The listing builds one solid part. Answer for the finished solid, in the listing's coordinates (mm). Face numbers are marked on the shaded views. Give positions to 0.01 mm unless a question says otherwise; leave off trailing zeros. Loops run counter-clockwise (first coordinate to the right, second up) from the corner with the lowest first, then second, coordinate; pieces in that order, holes last. Notation, with made-up numbers: M 36.25,-28.5 L 70.25,-28.5 A8 cw 70.25,-13.5 Z; hole C -17.75,35.25 d9. An arc over 180 degrees is marked long. One line per item, written item: value. Start each with the question number.
Q1. Flat-ended cylindrical pins translate along their axes: pin 1 (2 mm diameter, centred on x = 2, y = 2, fed in from +Z); pin 2 (4 mm diameter, centred on y = 5.5, z = 50.5, fed in from -X); pin 3 (4 mm diameter, centred on x = 5, z = 42, fed in from -Y); pin 4 (2 mm diameter, centred on y = 5.25, z = 51, fed in from -X). Find the tip coordinate at first contact, or state that the pin passes through.
Q2. The mould has two halves that part along X. Classify the marked faces 1, 2 and 3: +X half, -X half, draft (parallel to the pull), parting line (faces both ways), or undercut.
Q3. Consider L1, parallel to Z at x = 6.85, y = 5.25; L2, parallel to Z at x = 8, y = 2; L3, parallel to Y at x = 7.2, z = 91. Determine where each line is inside the solid, lowest interval first.
Q4. A cutting plane is placed at C-C, the plane z = 64.5. Determine the outline of the cut face in (x, y).
Q5. A cutting plane is placed at A-A, the plane z = 31. Determine the outline of the cut face in (x, y).
Q6. A cutting plane is placed at B-B, the plane x = 5.25. State how many separate pieces and enclosed holes the cut face has, and give its area (3 significant figures).
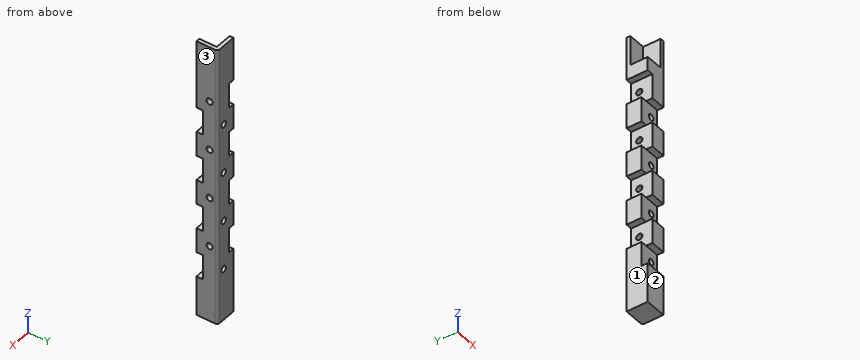
from build123d import *

# Parameters (mm, degrees)
SKETCH_W               = 8.5
SKETCH_H               = 8.5
PAD_DEPTH              = 113.5
SKETCH001_W            = 10
SKETCH001_H            = 10
POCKET_DEPTH           = 2.5
LINEARPATTERN_COUNT    = 4
LINEARPATTERN_PITCH    = 20
SKETCH002_W            = 10
SKETCH002_H            = 10
POCKET001_DEPTH        = 2.5
LINEARPATTERN001_COUNT = 4
LINEARPATTERN001_PITCH = 20
FILLET_R               = 1
SKETCH003_R            = 1.25
POCKET002_DEPTH        = 6.001
LINEARPATTERN002_COUNT = 4
LINEARPATTERN002_PITCH = 20
SKETCH004_R            = 1.25
POCKET003_DEPTH        = 6.001
LINEARPATTERN003_COUNT = 4
LINEARPATTERN003_PITCH = 20
SKETCH005_W            = 8.5
SKETCH005_H            = 8.5
POCKET004_DEPTH        = 12


with BuildPart() as part:
    # Sketch → Pad (new body)
    with BuildSketch(Plane.XY):
        with Locations((4.25, 4.25)):
            Rectangle(SKETCH_W, SKETCH_H)
    extrude(amount=PAD_DEPTH)

    # Sketch001 → Pocket (cut)
    with BuildSketch(Plane.XZ):
        with Locations((4.410969, 21)):
            Rectangle(SKETCH001_W, SKETCH001_H)
    pocket = extrude(amount=-POCKET_DEPTH, mode=Mode.SUBTRACT)

    # LinearPattern: Pocket ×4
    with Locations(*[(0, 0, i * LINEARPATTERN_PITCH) for i in range(1, LINEARPATTERN_COUNT)]):
        add(pocket, mode=Mode.SUBTRACT)

    # Sketch002 → Pocket001 (cut)
    with BuildSketch(Plane(origin=(0, 0, 0), x_dir=(0, -1, 0), z_dir=(-1, 0, 0))):
        with Locations((-4.326825, 31)):
            Rectangle(SKETCH002_W, SKETCH002_H)
    pocket001 = extrude(amount=-POCKET001_DEPTH, mode=Mode.SUBTRACT)

    # LinearPattern001: Pocket001 ×4
    with Locations(*[(0, 0, i * LINEARPATTERN001_PITCH) for i in range(1, LINEARPATTERN001_COUNT)]):
        add(pocket001, mode=Mode.SUBTRACT)

    # Fillet
    fillet_edges = [part.edges().sort_by_distance(p)[0] for p in [
        (8.5, 8.5, 56.75),
    ]]
    fillet(fillet_edges, radius=FILLET_R)

    # Sketch003 → Pocket002 (cut, through all)
    with BuildSketch(Plane.XZ.offset(-2.5)):
        with Locations((5.25, 21)):
            Circle(SKETCH003_R)
    pocket002 = extrude(amount=-POCKET002_DEPTH, mode=Mode.SUBTRACT)

    # LinearPattern002: Pocket002 ×4
    with Locations(*[(0, 0, i * LINEARPATTERN002_PITCH) for i in range(1, LINEARPATTERN002_COUNT)]):
        add(pocket002, mode=Mode.SUBTRACT)

    # Sketch004 → Pocket003 (cut, through all)
    with BuildSketch(Plane(origin=(2.5, 0, 0), x_dir=(0, -1, 0), z_dir=(-1, 0, 0))):
        with Locations((-5.25, 31)):
            Circle(SKETCH004_R)
    pocket003 = extrude(amount=-POCKET003_DEPTH, mode=Mode.SUBTRACT)

    # LinearPattern003: Pocket003 ×4
    with Locations(*[(0, 0, i * LINEARPATTERN003_PITCH) for i in range(1, LINEARPATTERN003_COUNT)]):
        add(pocket003, mode=Mode.SUBTRACT)

    # Sketch005 → Pocket004 (cut)
    with BuildSketch(Plane.XY.offset(113.5)):
        with Locations((2.75, 2.75)):
            Rectangle(SKETCH005_W, SKETCH005_H)
    extrude(amount=-POCKET004_DEPTH, mode=Mode.SUBTRACT)


solid = part.part
Answer block:
1. pin 1: z = 101.5
1. pin 2: x = 2.5
1. pin 3: y = 2.5
1. pin 4: through
2. face 1: -X half
2. face 2: draft
2. face 3: +X half
3. L1: 0 to 29.75, 32.25 to 49.75, 52.25 to 69.75, 72.25 to 89.75, 92.25 to 101.5
3. L2: 0 to 16, 26 to 36, 46 to 56, 66 to 76, 86 to 113.5
3. L3: 0 to 4, 6.5 to 8.5
4. outline: M 0,2.5 L 8.5,2.5 L 8.5,7.5 A1 ccw 7.5,8.5 L 0,8.5 Z
5. outline: M 2.5,0 L 8.5,0 L 8.5,4 L 2.5,4 Z; M 2.5,6.5 L 8.5,6.5 L 8.5,7.5 A1 ccw 7.5,8.5 L 2.5,8.5 Z
6. separate pieces: 5
6. enclosed holes: 4
6. area: 701 mm^2
